from build123d import *

# Parameters (mm, degrees)
F0_R     = 4.233333
F1_DEPTH = 2.794
F2_R     = 3.302
F3_DEPTH = 2.54
F4_SIZE  = 0.254


with BuildPart() as f1:
    # F0 (on Top) → F1 (new body)
    with BuildSketch(Plane.XY):
        Circle(F0_R)
    extrude(amount=F1_DEPTH)

    # F2 (on face) → F3 (cut)
    with BuildSketch(Plane.XY.offset(2.794)):
        Circle(F2_R)
    extrude(amount=-F3_DEPTH, mode=Mode.SUBTRACT)

    # F4
    f4_edges = [f1.edges().sort_by_distance(p)[0] for p in [
        (-4.233333, 0, 0),
    ]]
    chamfer(f4_edges, length=F4_SIZE)


solid = f1.part
Could you check a few things on this model? Use its own coordinates, in mm. A direction names the side the tool comes from. Coordinates: 2 decimals unless noted, no trailing zeros. Write each loop counter-clockwise with the first axis right and the second up, starting at its lowest first coordinate (ties: lowest second). Pieces come first, ordered by that corner, then holes. Notation, with made-up numbers: (83.5, -3) - (113.5, -3) arc R20 cw to (113.5, 31) - close; hole circle Ø7 at (84, -28). An arc over 180 degrees is marked (long way). Put each result on its own line as item: value. Start each with the question number.
Q1. Please list where these lines run through material, in increasing order: L1, parallel to Y at x = 0, z = 1.4; L2, parallel to Z at x = 0.5, y = 2; L3, parallel to X at y = 1, z = 1.9.
Q2. I want a section at C-C on z = 0.9. Write out the boundary of the cut face in (x, y), plus the area to 3 significant figures.
Q3. Which directions (+Z, -Z, +X, -X, +Y, -Y) give clear straight access to the entire face, cutting with the end or side of a thin tool? Please do faces 4 (the cylindrical face through (3.05, -1.26, 1.54)), 5 (the flat face through (0, 0, 0)).
Q4. Thinking about a two-plate mould opening in Y: for faces 1 (the flat face through (0, 0, 0.254)), 2 (the cylindrical face through (-0.918, -4.133, 1.506)), 3 (the flat face through (-3, -2, 2.794)), which applies, pulls with the +Y half, pulls with the -Y half, needs draft (parallel to the pull), parting line crosses it, or undercut?
Q5. I want a section at A-A on x = 0. Write out the boundary of the cut face in (y, z), plus the area to 3 significant figures.
Q6. I'm going to push flat-ended pins straight in: P1, Ø2, axis at x = 0, y = 0.5, coming from the +Z side; P2, Ø4, axis at x = -2.5, y = 2, coming from the -Z side. Where does each tip first touch, or does it pass through?
Checks:
1. L1: -4.23 to -3.3, 3.3 to 4.23
1. L2: 0 to 0.25
1. L3: -4.11 to -3.15, 3.15 to 4.11
2. outline: circle Ø8.47 at (0, 0); hole circle Ø6.6 at (0, 0)
2. area: 22.0 mm²
3. face 4: +Z
3. face 5: -Z, +X, -X, +Y, -Y
4. face 1: undercut
4. face 2: parting line crosses it
4. face 3: needs draft
5. outline: (-4.23, 0.25) - (-3.98, 0) - (3.98, 0) - (4.23, 0.25) - (4.23, 2.79) - (3.3, 2.79) - (3.3, 0.25) - (-3.3, 0.25) - (-3.3, 2.79) - (-4.23, 2.79) - close
5. area: 6.82 mm²
6. P1: z = 0.25
6. P2: z = 0
